For this review, take the finished solid that the model builds, in its own axes (mm). Face numbers are marked on the shaded views. A direction names the side the tool comes from. Round coordinates to 2 decimals unless told otherwise and drop trailing zeros. Order: outer loops, then holes, each group sorted by start corner. A loop starts at its lowest first (then second) coordinate and runs counter-clockwise, first axis right, second up. Notation, with made-up numbers: (65, 10.25) - (76, 10.25) arc R26 cw to (76, 45.25) - close; hole circle Ø7 at (12, -37). An arc over 180 degrees is marked (long way). One line per question, with ' | ' between items.
```python
from build123d import *

# Parameters (mm, degrees)
SKETCH_1_R          = 38
EXTRUDE_1_DEPTH     = 150
SKETCH_2_R          = 10
EXTRUDE_2_DEPTH     = 66
SKETCH_3_R          = 7.5
EXTRUDE_3_DEPTH     = 22
CUT_EXTRUDE_START   = 7.5
CUT_EXTRUDE_1_DEPTH = 3


with BuildPart() as part:
    # 草图1 → 凸台-拉伸1 (new, symmetric)
    with BuildSketch(Plane.XY):
        Circle(SKETCH_1_R)
    extrude(amount=EXTRUDE_1_DEPTH, both=True)

    # 草图2 → 凸台-拉伸2 (add)
    with BuildSketch(Plane.XY.offset(150)):
        Circle(SKETCH_2_R)
    extrude_2 = extrude(amount=EXTRUDE_2_DEPTH)

    # 镜向1: 凸台-拉伸2 across plane
    add(extrude_2.mirror(Plane.XY))

    # 草图3 → 凸台-拉伸3 (add)
    with BuildSketch(Plane.XY.offset(216)):
        Circle(SKETCH_3_R)
    extrude(amount=EXTRUDE_3_DEPTH)

    # 草图4 → 切除-拉伸1 (cut)
    with BuildSketch(Plane(origin=(0, 0, 0), x_dir=(1, 0, 0), z_dir=(0, 1, 0)).offset(CUT_EXTRUDE_START)):
        with BuildLine():
            Line((-2.5, -238), (-2.5, -223))
            ThreePointArc((-2.5, -223), (0, -220.5), (2.5, -223))
            Line((2.5, -223), (2.5, -238))
            ThreePointArc((2.5, -238), (0, -240.5), (-2.5, -238))
        make_face()
    extrude(amount=-CUT_EXTRUDE_1_DEPTH, mode=Mode.SUBTRACT)


solid = part.part
```
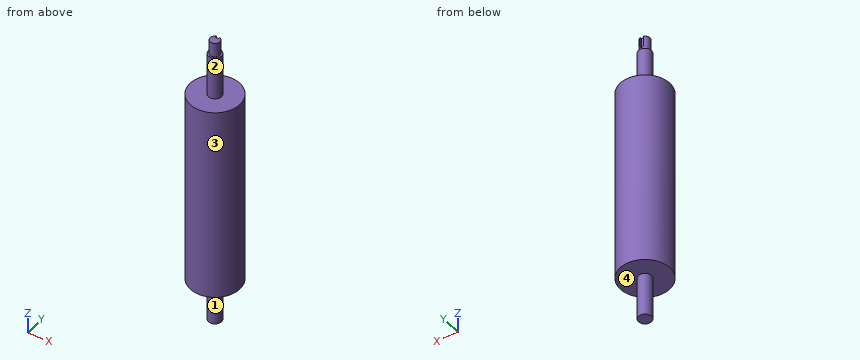
(1) We need section C-C on x = -20. State the section outline as (y, z) points.
Output values:
outline: (-32.31, -150) - (32.31, -150) - (32.31, 150) - (-32.31, 150) - close
(2) We need section D-D on z = 30. State the section outline as (x, y) points, plus the area to 3 significant figures.
Output values:
outline: circle Ø76 at (0, 0) | area: 4,540 mm^2
(3) For the marked faces 1 and 2, list the 3-axis set-ups (+Z, -Z, +X, -X, +Y, -Y) from which the entire face can be reached by the end or side of a thin tool; tool diameter is ignored.
Output values:
face 1: -Z | face 2: +Z
(4) We need section B-B on z = 191. State the section outline as (x, y) points.
Output values:
outline: circle Ø20 at (0, 0)
(5) For probe 1 along Z at (x, y) = (-1.5, -34); probe 2 along Y at (x, z) = (15, -79); probe 3 along Y at (x, z) = (-14.5, 119), list the stretches that pass through material, from the lowest coordinate up. Write a range as [from, to].
Output values:
probe 1: [-150, 150] | probe 2: [-34.91, 34.91] | probe 3: [-35.12, 35.12]
(6) We need section A-A on y = 0. State the section outline as (x, z) points, plus the area to 3 significant figures.
Output values:
outline: (-38, -150) - (-10, -150) - (-10, -216) - (10, -216) - (10, -150) - (38, -150) - (38, 150) - (10, 150) - (10, 216) - (7.5, 216) - (7.5, 238) - (-7.5, 238) - (-7.5, 216) - (-10, 216) - (-10, 150) - (-38, 150) - close | area: 25,800 mm^2
(7) Insertion check: pin 1 (1 mm diameter, centred on x = 17.5, z = 129, fed in from +Y); pin 2 (5.5 mm diameter, centred on x = 1, z = 229.5, fed in from +Y); pin 3 (0.8 mm diameter, centred on y = 6.5, z = 228.5, fed in from -X). Each pin has a flat end and moves straight along its axis. Give the tip position at first contact, or say it passes through.
Output values:
pin 1: y = 33.99 | pin 2: y = 7.07 | pin 3: x = -4.36
(8) Mouldability with a two-part tool opening along Y and no side actions: class the marked faces 3 and 4 as released by +Y, released by -Y, zero draft, split by the parting line, or undercut.
Output values:
face 3: split by the parting line | face 4: zero draft
